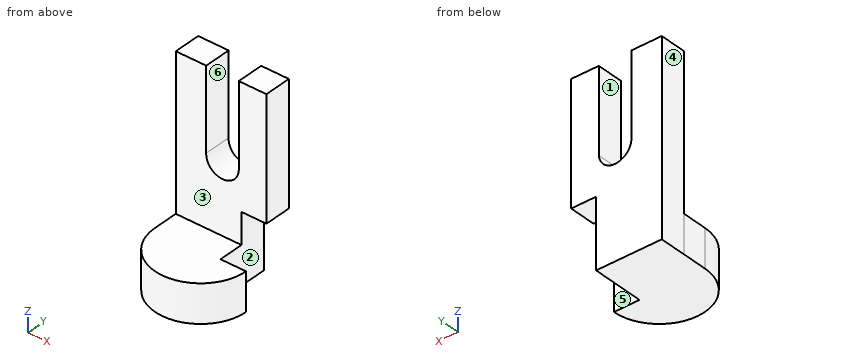
from build123d import *

# Parameters (mm, degrees)
F1_DEPTH  = 25.4
F2_W      = 60.9679538757
F2_H      = 16.9523619115
F3_DEPTH  = 25.4
F4_W      = 17.1053176746
F4_H      = 16.9523619115
F5_DEPTH  = 25.4
F6_W      = 60.6785267591
F6_H      = 17.9788209498
F7_DEPTH  = 127
F8_W      = 16.7008666322
F8_H      = 20.6584424436
F8_H_2    = 25.4
F9_DEPTH  = 25.4
F11_DEPTH = 25.4


with BuildPart() as f1:
    # F0 (on Top) → F1 (new body)
    with BuildSketch(Plane.XY):
        with BuildLine():
            Line((29.8158377409, 0), (-31.3191562891, 0))
            ThreePointArc((-31.3191562891, 0), (-0.7516592741, -30.4326055801), (29.8158377409, 0))
        make_face()
    extrude(amount=F1_DEPTH)

    # F2 (on Top) → F3 (join)
    with BuildSketch(Plane.XY):
        with Locations((-0.8351793513, 8.4761809558)):
            Rectangle(F2_W, F2_H)
    extrude(amount=F3_DEPTH)

    # F4 (on face) → F5 (cut)
    with BuildSketch(Plane.XY.offset(25.4)):
        with Locations((21.2631789036, 8.4761809558)):
            Rectangle(F4_W, F4_H)
    extrude(amount=-F5_DEPTH, mode=Mode.SUBTRACT)

    # F6 (on Top) → F7 (join)
    with BuildSketch(Plane.XY):
        with Locations((-0.9278766811, 25.8058961481)):
            Rectangle(F6_W, F6_H)
    extrude(amount=F7_DEPTH)

    # F8 (on face) → F9 (cut)
    with BuildSketch(Plane.XZ.offset(-16.8164856732)):
        with Locations((21.0609533824, 35.7292212218)):
            Rectangle(F8_W, F8_H)
        with Locations((21.0609533824, 12.7)):
            Rectangle(F8_W, F8_H_2)
    extrude(amount=-F9_DEPTH, mode=Mode.SUBTRACT)

    # F10 (on face) → F11 (cut)
    with BuildSketch(Plane.XZ.offset(-16.8164856732)):
        with BuildLine():
            Line((-10.910176672, 127), (-10.910176672, 72.342030704))
            ThreePointArc((-10.910176672, 72.342030704), (-0.6730834345, 60.9522454092), (10.8875039349, 70.9960547807))
            Line((10.8875039349, 70.9960547807), (10.8875039349, 127))
            Line((10.8875039349, 127), (-10.910176672, 127))
        make_face()
    extrude(amount=-F11_DEPTH, mode=Mode.SUBTRACT)


solid = f1.part
Geometry: final body of the model. Coordinates: model frame, mm. Face numbers are marked on the shaded views. A direction names the side the tool comes from. Coordinates: 2 decimals unless noted, no trailing zeros. Loops run counter-clockwise (first coordinate to the right, second up) from the corner with the lowest first, then second, coordinate; pieces in that order, holes last. Notation, with made-up numbers: (-13, 51) - (-8, 51) arc R21 ccw to (-8, 62) - close; hole circle Ø9 at (-4, 45). An arc over 180 degrees is marked (long way). One line per question, with ' | ' between items. Start each with the question number.
(1) Cut plane B-B on x = 14. Output: boundary loops of the cut face in (y, z), and give its area (3 significant figures).
(2) First-contact query: pin 1 (1.5 mm diameter, centred on x = 6.5, y = 27, fed in from +Z); pin 2 (1 mm diameter, centred on x = 10.5, y = 8, fed in from -Z); pin 3 (10 mm diameter, centred on y = 26, z = 87, fed in from -X); pin 4 (8.5 mm diameter, centred on x = 21.5, z = 14.5, fed in from +Y). Flat tips, straight axial feed; report the tip coordinate or a pass-through.
(3) Draft query along X for the marked faces 4, 5 and 6. Return one class per face: +X half, -X half, draft (parallel to the pull), parting line (faces both ways), or undercut.
(4) Cut plane D-D on z = 16.5. Output: boundary loops of the cut face in (x, y).
(5) Ray query, L1, parallel to X at y = 21, z = 96; L2, parallel to Z at x = 27.5, y = -6; L3, parallel to Y at x = -18, z = 77. Return the intervals inside material, ascending. Write a range as from..to.
(6) Reachability of the marked faces 1, 2 and 3 from +Z, -Z, +X, -X, +Y, -Y: full face, straight path, thin tool, end or side. Return the list, or none.
(7) Cut plane A-A on z = 75.5. Output: boundary loops of the cut face in (x, y), and give its area (3 significant figures).
(8) Cut plane C-C on y = 22. Output: boundary loops of the cut face in (x, z).
Here are the results:
1) outline: (-26.64, 0) - (0, 0) - (0, 25.4) - (-26.64, 25.4) - close; (16.82, 46.06) - (34.8, 46.06) - (34.8, 127) - (16.82, 127) - close | area: 2,130 mm²
2) pin 1: z = 63.69 | pin 2: z = 0 | pin 3: x = -31.27 | pin 4: y = 0
3) face 4: -X half | face 5: draft | face 6: undercut
4) outline: (-31.32, 0) arc R30.57 ccw to (29.82, 0) - (12.71, 0) - (12.71, 34.8) - (-31.27, 34.8) - (-31.27, 16.95) - (-31.32, 16.95) - close
5) L1: -31.27..-10.91, 10.89..29.41 | L2: 0..25.4 | L3: 16.82..34.8
6) face 1: +Z, +Y, -Y | face 2: -Z, +X, +Y | face 3: +Z, +X, -X, -Y
7) outline: (-31.27, 16.82) - (-10.91, 16.82) - (-10.91, 34.8) - (-31.27, 34.8) - close; (10.89, 16.82) - (29.41, 16.82) - (29.41, 34.8) - (10.89, 34.8) - close | area: 699 mm²
8) outline: (-31.27, 0) - (12.71, 0) - (12.71, 46.06) - (29.41, 46.06) - (29.41, 127) - (10.89, 127) - (10.89, 71) arc R10.92 cw to (-10.91, 72.34) - (-10.91, 127) - (-31.27, 127) - close
